The figure shows three views and two pictorial views of one solid part (mm, origin at its lowest corner). Answer the questions. A direction names the side the tool comes from. Coordinates: 2 decimals unless noted, no trailing zeros. Write each loop counter-clockwise with the first axis right and the second up, starting at its lowest first coordinate (ties: lowest second). Pieces come first, ordered by that corner, then holes.
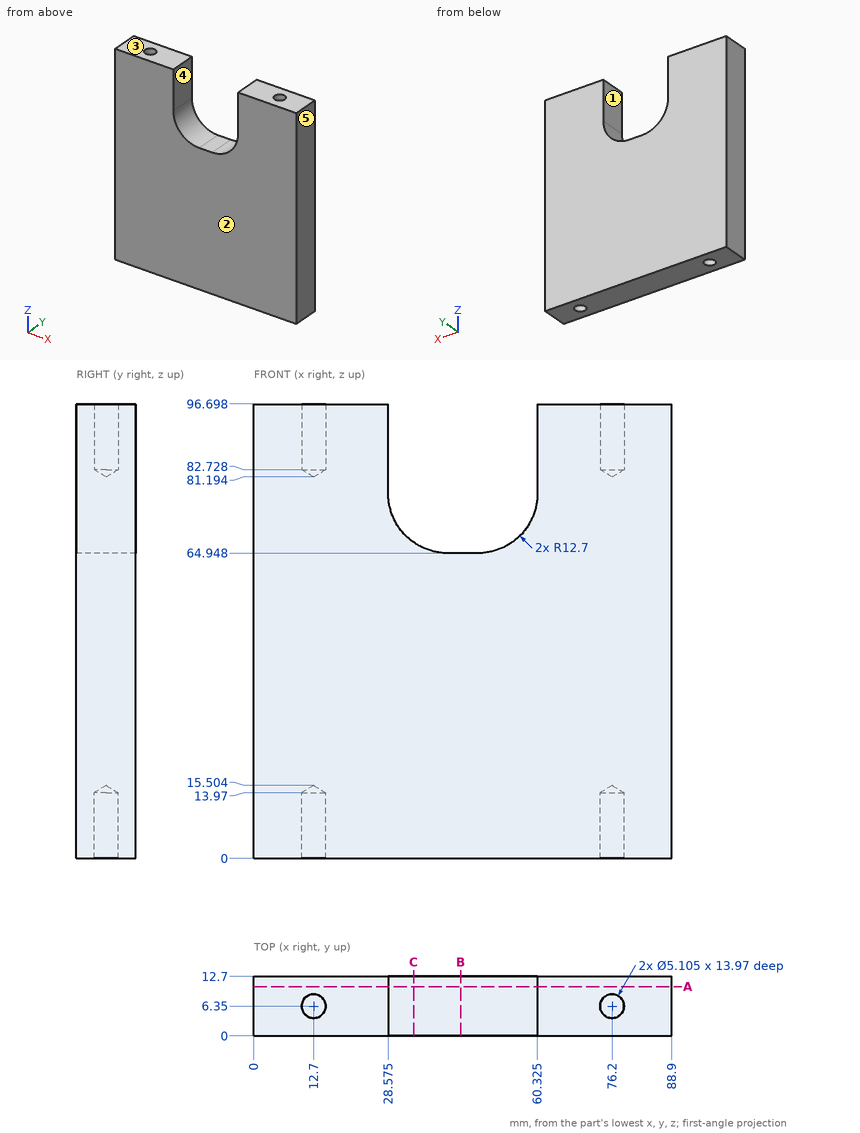
1. Flat-ended cylindrical pins translate along their axes: P1, Ø4.5, axis at x = 76.2, y = 6.35, coming from the +Z side (1 decimal); P2, Ø4.5, axis at x = 12.7, y = 6.35, coming from the -Z side; P3, Ø1.9, axis at x = 43.5, y = 5, coming from the +Z side. Find the tip coordinate at first contact, or state that the pin passes through.
Results found:
P1: stops at z = 82.5
P2: stops at z = 14.15
P3: stops at z = 64.95
2. Section C-C on x = 34 is taken. Give the vertices of the cut face in (y, z), then the cut area to 3 significant figures.
Results found:
outline: (0, 0) - (12.7, 0) - (12.7, 67.24) - (0, 67.24) - close
area: 854 mm2
3. Find the intervals of material crossed by L1, parallel to X at y = 6.35, z = 92 (1 decimal); L2, parallel to Y at x = 12.7, z = 7.5; L3, parallel to X at y = 1.5, z = 85 (1 decimal), in increasing order.
Results found:
L1: x = 0 to 10.1, 15.3 to 28.6, 60.3 to 73.6, 78.8 to 88.9
L2: y = 0 to 3.8, 8.9 to 12.7
L3: x = 0 to 28.6, 60.3 to 88.9
4. Section B-B on x = 44 is taken. Give the vertices of the cut face in (y, z), then the cut area to 3 significant figures.
Results found:
outline: (0, 0) - (12.7, 0) - (12.7, 64.95) - (0, 64.95) - close
area: 825 mm2
5. A tool of negligible diameter and unlimited length cuts with its end or side. For the marked faces 1 and 2, from which of +Z, -Z, +X, -X, +Y, -Y can it reach the whole face along a straight path? Write none if from no direction.
Results found:
face 1: +Z, +Y, -Y
face 2: +Z, -Z, +X, -X, -Y
6. For a pull along X with two mould halves and no side action, classify the marked faces 3, 4 and 5 as pulls with the +X half, pulls with the -X half, needs draft (parallel to the pull), parting line crosses it, or undercut.
Results found:
face 3: needs draft
face 4: undercut
face 5: pulls with the +X half
7. Section A-A on y = 10.5 is taken. Give the vertices of the cut face in (x, z) (1 decimal), then the cut area to 3 significant figures.
Results found:
outline: (0, 0) - (88.9, 0) - (88.9, 96.7) - (60.3, 96.7) - (60.3, 77.6) arc R12.7 cw to (47.6, 64.9) - (41.3, 64.9) arc R12.7 cw to (28.6, 77.6) - (28.6, 96.7) - (0, 96.7) - close
area: 7,660 mm2
